Geometry check sheet. Reference: drawing and pictorial views, mm from the part's lowest x, y, z. A direction names the side the tool comes from. Give positions to 0.01 mm unless a question says otherwise; leave off trailing zeros. Order: outer loops, then holes, each group sorted by start corner. A loop starts at its lowest first (then second) coordinate and runs counter-clockwise, first axis right, second up. Notation, with made-up numbers: (-6.75, -2.5) - (34.25, -2.5) arc R35 ccw to (34.25, 34.5) - close; hole circle Ø9 at (-0.5, -4). An arc over 180 degrees is marked (long way). Answer as a JSON object with one key per item and string values.
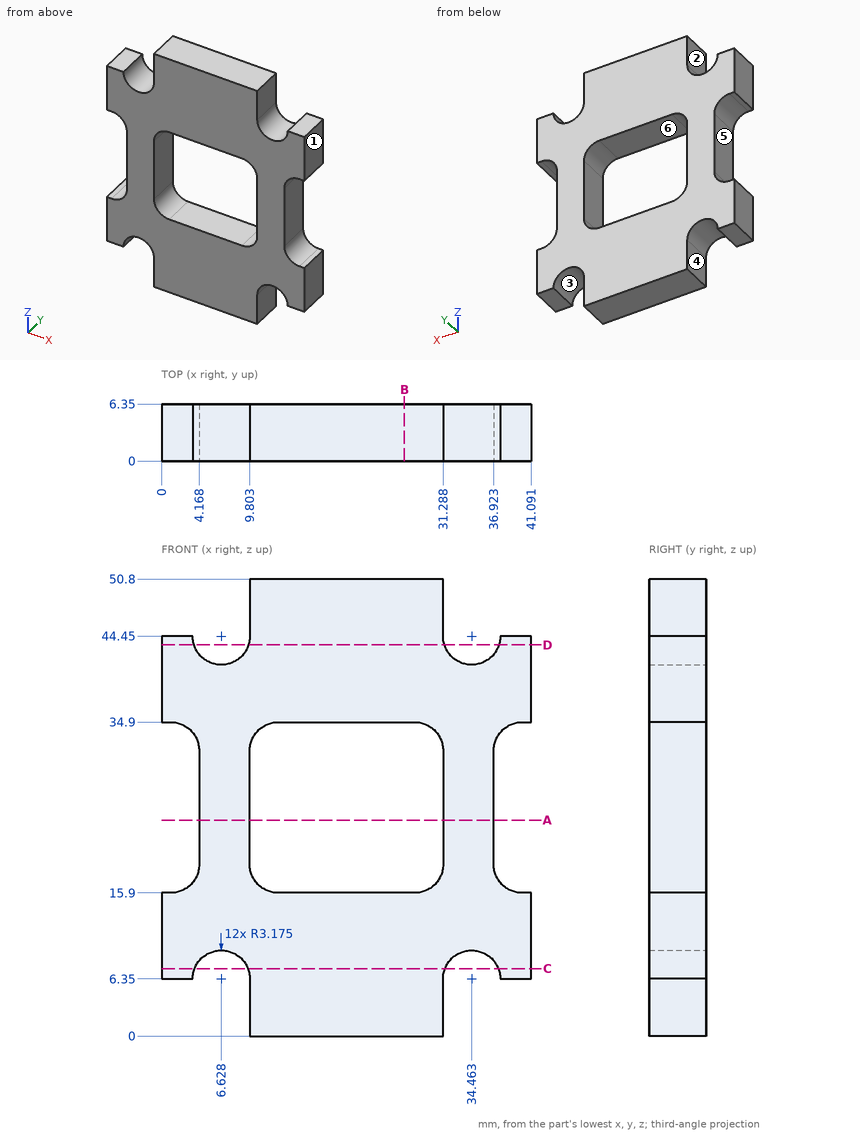
(1) Release check for a two-part mould opening along X. For the marked faces 1, 2 and 3 record: pulls with the +X half, pulls with the -X half, needs draft (parallel to the pull), parting line crosses it, or undercut.
Computed values:
{"face 1": "pulls with the +X half", "face 2": "pulls with the -X half", "face 3": "undercut"}
(2) Material ranges on line 1 along Z through (x, y) = (17, 2); line 2 along X through (y, z) = (4.25, 31); line 3 along X through (y, z) = (1, 7) (1 decimal), recorded low to high. Write a range as [from, to].
Computed values:
{"line 1": "z = [0, 15.9], [34.9, 50.8]", "line 2": "x = [4.17, 9.8], [31.29, 36.92]", "line 3": "x = [0, 3.5], [9.7, 31.4], [37.6, 41.1]"}
(3) Gauge pin test, flat ends, axial feed: pin 1 Ø1.7 at (x, y) = (1.5, 2.5) entering from +Z; pin 2 Ø3 at (y, z) = (4, 23.5) entering from +X; pin 3 Ø3 at (y, z) = (2, 46) entering from -X. Record the tip position at first contact, or that the pin passes through.
Computed values:
{"pin 1": "stops at z = 44.45", "pin 2": "stops at x = 36.92", "pin 3": "stops at x = 9.8"}
(4) Section check A-A (z = 24). Record the cut outline in (x, y).
Computed values:
{"outline": "(4.17, 0) - (9.8, 0) - (9.8, 6.35) - (4.17, 6.35) - close; (31.29, 0) - (36.92, 0) - (36.92, 6.35) - (31.29, 6.35) - close"}
(5) Section check C-C (z = 7.5). Record the cut outline in (x, y), then the cut area to 3 significant figures.
Computed values:
{"outline": "(0, 0) - (3.67, 0) - (3.67, 6.35) - (0, 6.35) - close; (9.59, 0) - (31.5, 0) - (31.5, 6.35) - (9.59, 6.35) - close; (37.42, 0) - (41.09, 0) - (41.09, 6.35) - (37.42, 6.35) - close", "area": "186 mm²"}
(6) Section check B-B (x = 27). Record the cut outline in (y, z).
Computed values:
{"outline": "(0, 0) - (6.35, 0) - (6.35, 15.9) - (0, 15.9) - close; (0, 34.9) - (6.35, 34.9) - (6.35, 50.8) - (0, 50.8) - close"}
(7) Section check D-D (z = 43.5). Record the cut outline in (x, y), then the cut area to 3 significant figures.
Computed values:
{"outline": "(0, 0) - (3.6, 0) - (3.6, 6.35) - (0, 6.35) - close; (9.66, 0) - (31.43, 0) - (31.43, 6.35) - (9.66, 6.35) - close; (37.49, 0) - (41.09, 0) - (41.09, 6.35) - (37.49, 6.35) - close", "area": "184 mm²"}
(8) Access from +Z, -Z, +X, -X, +Y, -Y to the whole of each face (thin tool, end or side, straight path). Record for the marked faces 4, 5 and 6.
Computed values:
{"face 4": "-Z, -X, +Y, -Y", "face 5": "-X, +Y, -Y", "face 6": "+Y, -Y"}
